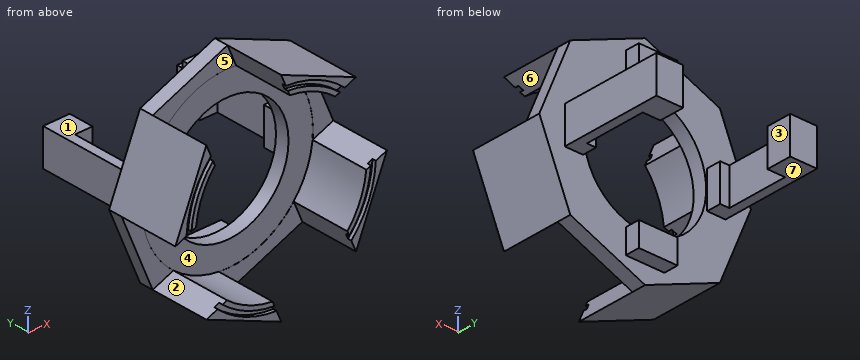
from build123d import *

# Parameters (mm, degrees)
BOSS_EXTRUDE1_DEPTH = 7.61
SKETCH5_R           = 17.78
CUT_EXTRUDE2_DEPTH  = 12.3444
SKETCH6_R           = 12.7
CUT_EXTRUDE3_DEPTH  = 3.8756
SKETCH7_W           = 16.833639174
SKETCH7_H           = 12.3244
CUT_EXTRUDE4_DEPTH  = 50.056819587
SKETCH8_W           = 16.833639174
SKETCH8_H           = 12.3244
CUT_EXTRUDE5_DEPTH  = 50.056819587
SKETCH10_R          = 19.69527877
SKETCH10_R_2        = 18.703643049
CUT_EXTRUDE7_DEPTH  = 0.762
SKETCH11_W          = 3.81
SKETCH11_H          = 7.62
BOSS_EXTRUDE2_DEPTH = 21.02
SKETCH13_W          = 29.591
SKETCH13_H          = 7.62
CUT_EXTRUDE8_DEPTH  = 18.02
SKETCH15_W          = 8.037943886
SKETCH15_H          = 5
BOSS_EXTRUDE3_DEPTH = 3
SKETCH16_W          = 7.62
SKETCH16_H          = 5.23
BOSS_EXTRUDE4_DEPTH = 3.67


with BuildPart() as part:
    # Sketch1 → Boss-Extrude1 (new body, symmetric)
    with BuildSketch(Plane(origin=(0, 0, 0), x_dir=(1, 0, 0), z_dir=(0, 1, 0))):
        Polygon((21.99420951, 0), (15.552254691, 15.552254691), (0, 21.99420951), (-15.552254691, 15.552254691), (-21.99420951, 0), (-15.552254691, -15.552254691), (0, -21.99420951), (15.552254691, -15.552254691), align=None)
    extrude(amount=BOSS_EXTRUDE1_DEPTH, both=True)

    # Sketch5 → Cut-Extrude2 (cut)
    with BuildSketch(Plane.XZ.offset(7.61)):
        Circle(SKETCH5_R)
    extrude(amount=-CUT_EXTRUDE2_DEPTH, mode=Mode.SUBTRACT)

    # Sketch6 → Cut-Extrude3 (cut, through all)
    with BuildSketch(Plane.XZ.offset(-4.7344)):
        Circle(SKETCH6_R)
    extrude(amount=-CUT_EXTRUDE3_DEPTH, mode=Mode.SUBTRACT)

    # Sketch7 → Cut-Extrude4 (cut, through all)
    with BuildSketch(Plane(origin=(-7.776127346, 0, 18.773232101), x_dir=(0.923879533, 0, 0.382683432), z_dir=(-0.382683432, 0, 0.923879533))):
        with Locations((0, -1.4478)):
            Rectangle(SKETCH7_W, SKETCH7_H)
    extrude(amount=-CUT_EXTRUDE4_DEPTH, mode=Mode.SUBTRACT)

    # Sketch8 → Cut-Extrude5 (cut, through all)
    with BuildSketch(Plane(origin=(18.773232101, 0, 7.776127346), x_dir=(0.382683432, 0, -0.923879533), z_dir=(0.923879533, 0, 0.382683432))):
        with Locations((0, -1.4478)):
            Rectangle(SKETCH8_W, SKETCH8_H)
    extrude(amount=-CUT_EXTRUDE5_DEPTH, mode=Mode.SUBTRACT)

    # Sketch10 → Cut-Extrude7 (cut)
    with BuildSketch(Plane.XZ.offset(7.61)):
        Circle(SKETCH10_R)
        Circle(SKETCH10_R_2, mode=Mode.SUBTRACT)
    extrude(amount=-CUT_EXTRUDE7_DEPTH, mode=Mode.SUBTRACT)

    # Sketch11 → Boss-Extrude2 (add)
    with BuildSketch(Plane(origin=(0, 7.61, 0), x_dir=(1, 0, 0), z_dir=(0, 1, 0))):
        with Locations((14.7955, 0)):
            Rectangle(SKETCH11_W, SKETCH11_H)
        with Locations((-14.7955, 0)):
            Rectangle(SKETCH11_W, SKETCH11_H)
    extrude(amount=BOSS_EXTRUDE2_DEPTH)

    # Sketch13 → Cut-Extrude8 (cut)
    with BuildSketch(Plane(origin=(0, 28.63, 0), x_dir=(1, 0, 0), z_dir=(0, 1, 0))):
        Rectangle(SKETCH13_W, SKETCH13_H)
    extrude(amount=-CUT_EXTRUDE8_DEPTH, mode=Mode.SUBTRACT)

    # Sketch15 → Boss-Extrude3 (add)
    with BuildSketch(Plane(origin=(0, 7.61, 0), x_dir=(1, 0, 0), z_dir=(0, 1, 0))):
        with Locations((0, -15.75)):
            Rectangle(SKETCH15_W, SKETCH15_H)
        with Locations((0, 15.75)):
            Rectangle(SKETCH15_W, SKETCH15_H)
    extrude(amount=BOSS_EXTRUDE3_DEPTH)

    # Sketch16 → Boss-Extrude4 (add)
    with BuildSketch(Plane(origin=(-14.7955, 0, 0), x_dir=(0, 0, -1), z_dir=(1, 0, 0))):
        with Locations((0, 26.015)):
            Rectangle(SKETCH16_W, SKETCH16_H)
    boss_extrude4 = extrude(amount=BOSS_EXTRUDE4_DEPTH)

    # Mirror1: Boss-Extrude4 across plane
    add(boss_extrude4.mirror(Plane(origin=(0, 0, 0), x_dir=(0, 0, 1), z_dir=(1, 0, 0))))


solid = part.part
Input: part model. Units: mm. Frame: model coordinates. Face numbers are marked on the shaded views. A direction names the side the tool comes from. Round coordinates to 2 decimals unless told otherwise and drop trailing zeros. Order: outer loops, then holes, each group sorted by start corner. A loop starts at its lowest first (then second) coordinate and runs counter-clockwise, first axis right, second up.
1. Mould query, pull axis Z, two halves, no side actions, for the marked faces 5, 6 and 7. Classes: released by +Z, released by -Z, zero draft, split by the parting line, or undercut.
The answers:
face 5: zero draft
face 6: undercut
face 7: released by -Z
2. Set-up query: the marked faces 1, 2, 3 and 4. Return all of +Z, -Z, +X, -X, +Y, -Y with unobstructed straight access to the full face (end or side cutting, diameter ignored); none if empty.
The answers:
face 1: +Z, +X, -X, +Y
face 2: -X, -Y
face 3: +Z, -Z, +Y, -Y
face 4: -Y
3. Material intervals for line 1 (Z direction, x = 0, y = 5); line 2 (X direction, y = 19.5, z = 0.5); line 3 (Y direction, x = -12, z = 3), sorted ascending.
The answers:
line 1: z = -21.99 to -12.7, 12.7 to 21.99
line 2: x = -16.7 to -14.8, 14.8 to 16.7
line 3: y = 23.4 to 28.63
4. Cut plane A-A, the plane y = 18.5. Output: boundary loops of the cut face in (x, z).
The answers:
outline: (-16.7, -3.81) - (-14.8, -3.81) - (-14.8, 3.81) - (-16.7, 3.81) - close; (14.8, -3.81) - (16.7, -3.81) - (16.7, 3.81) - (14.8, 3.81) - close
5. Pin query (flat end, axial travel): P1, Ø4, axis at x = -16.5, y = 8.5, coming from the -Z side; P2, Ø1.5, axis at y = 8.5, z = 14.5, coming from the -X side; P3, Ø1.6, axis at y = 27, z = 0.5, coming from the +X side. Return the tip coordinate at first contact, or that it passes through.
The answers:
P1: stops at z = -15.9
P2: stops at x = -4.02
P3: stops at x = 16.7
